Part model, mm, in its own coordinate system. Round coordinates to 2 decimals unless told otherwise and drop trailing zeros. Order: outer loops, then holes, each group sorted by start corner. A loop starts at its lowest first (then second) coordinate and runs counter-clockwise, first axis right, second up. Notation, with made-up numbers: (83.25, -3) - (140.25, -3) arc R22 ccw to (140.25, 15) - close; hole circle Ø2 at (-23, -8). An arc over 180 degrees is marked (long way). Return JSON: item names as keys, results as strings. Group by question number.
Item 1: Probe probe 1 along X at (y, z) = (3, -20); probe 2 along X at (y, z) = (3.75, 18); probe 3 along X at (y, z) = (3.25, 0). List the from-to ranges inside material, lowest first.
Item 2: Drop flat-ended pins along their axis: pin 1 (1.5 mm diameter, centred on y = 4.5, z = 18.5, fed in from +X); pin 2 (7 mm diameter, centred on x = -33.17, z = -45.65, fed in from +Y); pin 3 (1 mm diameter, centred on x = 2, y = 5, fed in from -Z). Give the stop position or say it passes through.
Item 3: Saw through at C-C on y = 3.25. State how many separate pieces and enclosed holes the cut face has, and give its area (3 significant figures).
Item 4: Saw through at B-B on x = 0. List the corners of the cut face in (y, z).
Item 5: Saw through at A-A on z = 0. List the corners of the cut face in (x, y), and give its area (3 significant figures).
Item 6: Saw through at D-D on x = 16. List the corners of the cut face in (y, z).
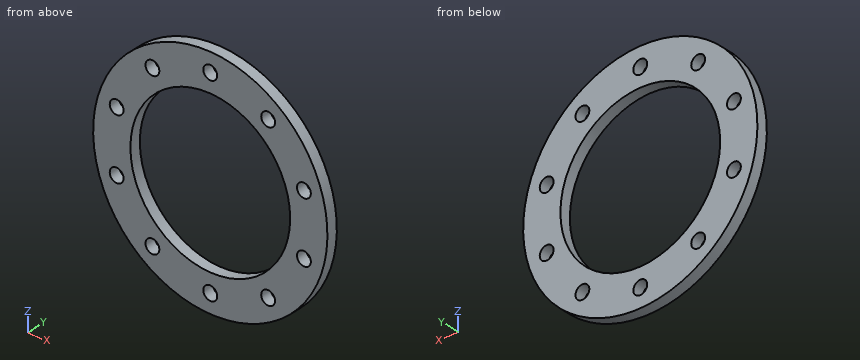
```python
from build123d import *

# Parameters (mm, degrees)
SKETCH1_R           = 67.133194764
SKETCH1_R_2         = 45.789019651
BOSS_EXTRUDE1_DEPTH = 6.35
CUT_EXTRUDE1_REACH  = 97.153
SKETCH2_R           = 3.96875
CIRPATTERN1_COUNT   = 10


with BuildPart() as part:
    # Sketch1 → Boss-Extrude1 (new body)
    with BuildSketch(Plane(origin=(0, 0, 0), x_dir=(1, 0, 0), z_dir=(0, 1, 0))):
        with Locations(Location((0, 0, 0), (0, 0, 270))):
            Circle(SKETCH1_R)
        with Locations(Location((0, 0, 0), (0, 0, 270))):
            Circle(SKETCH1_R_2, mode=Mode.SUBTRACT)
    extrude(amount=BOSS_EXTRUDE1_DEPTH)

    # Sketch2 → Cut-Extrude1 (cut, up to next)
    with BuildSketch(Plane(origin=(0, 6.35, 0), x_dir=(1, 0, 0), z_dir=(0, 1, 0)), mode=Mode.PRIVATE) as cut_extrude1_sk1:
        with Locations(Location((0, 56.428647919, 0), (0, 0, 270))):
            Circle(SKETCH2_R)
    cut_extrude1_tool1 = extrude(cut_extrude1_sk1.sketch, amount=-CUT_EXTRUDE1_REACH, mode=Mode.PRIVATE) & part.part
    cut_extrude1 = cut_extrude1_tool1.solids().sort_by_distance((0, 6.35, -56.428648))[0]
    add(cut_extrude1, mode=Mode.SUBTRACT)

    # CirPattern1: Cut-Extrude1 ×10 about axis
    cirpattern1_axis = Axis((0, 0, 0), (0, 1, 0))
    for i in range(1, CIRPATTERN1_COUNT):
        add(cut_extrude1.rotate(cirpattern1_axis, i * 360 / CIRPATTERN1_COUNT), mode=Mode.SUBTRACT)


solid = part.part
```
Filled in:
{
 "1": {"probe 1": "x = -64.08 to -56.7, -50.64 to -41.19, 41.19 to 50.64, 56.7 to 64.08", "probe 2": "x = -64.68 to -57.6, -49.74 to -42.1, 42.1 to 49.74, 57.6 to 64.68", "probe 3": "x = -67.13 to -45.79, 45.79 to 67.13"},
 "2": {"pin 1": "stops at x = 64.74", "pin 2": "passes through", "pin 3": "stops at z = -67.12"},
 "3": {"separate pieces": "1", "enclosed holes": "11", "area": "7,080 mm^2"},
 "4": {"outline": "(0, -67.13) - (6.35, -67.13) - (6.35, -60.4) - (0, -60.4) - close; (0, -52.46) - (6.35, -52.46) - (6.35, -45.79) - (0, -45.79) - close; (0, 45.79) - (6.35, 45.79) - (6.35, 52.46) - (0, 52.46) - close; (0, 60.4) - (6.35, 60.4) - (6.35, 67.13) - (0, 67.13) - close"},
 "5": {"outline": "(-67.13, 0) - (-45.79, 0) - (-45.79, 6.35) - (-67.13, 6.35) - close; (45.79, 0) - (67.13, 0) - (67.13, 6.35) - (45.79, 6.35) - close", "area": "271 mm^2"},
 "6": {"outline": "(0, -65.2) - (6.35, -65.2) - (6.35, -42.9) - (0, -42.9) - close; (0, 42.9) - (6.35, 42.9) - (6.35, 65.2) - (0, 65.2) - close"}
}
